```python
from build123d import *

# Parameters (mm, degrees)
SKETCH023_W  = 3.3
SKETCH023_H  = 2.2
PAD017_DEPTH = 2.5
PAD016_DEPTH = 5.5
FILLET001_R  = 1.1


with BuildPart() as pad_button_hole:
    # Sketch023 → Pad017 (new body)
    with BuildSketch(Plane.XY):
        Rectangle(SKETCH023_W, SKETCH023_H)
    extrude(amount=PAD017_DEPTH)


with BuildPart() as cut_button_small_final:
    # Sketch020 → Pad016 (new body)
    with BuildSketch(Plane.XY):
        with BuildLine():
            ThreePointArc((4.169285, 2.5), (0, 2.670418), (-4.169285, 2.5))
            ThreePointArc((-4.169285, 2.5), (-5.113877, 2.040693), (-5.5, 1.0639))
            ThreePointArc((-5.5, 1.0639), (-5.502959, 0), (-5.5, -1.0639))
            ThreePointArc((-5.5, -1.0639), (-5.113877, -2.040693), (-4.169285, -2.5))
            ThreePointArc((-4.169285, -2.5), (0, -2.670418), (4.169285, -2.5))
            ThreePointArc((4.169285, -2.5), (5.113877, -2.040693), (5.5, -1.0639))
            ThreePointArc((5.5, -1.0639), (5.502959, 0), (5.5, 1.0639))
            ThreePointArc((5.5, 1.0639), (5.113877, 2.040693), (4.169285, 2.5))
        make_face()
    extrude(amount=PAD016_DEPTH)

    # Fillet001
    fillet001_edges = [cut_button_small_final.edges().sort_by_distance(p)[0] for p in [
        (0, 2.670418, 5.5),
        (-5.113877, 2.040693, 5.5),
        (-5.502959, 0, 5.5),
        (-5.113877, -2.040693, 5.5),
        (0, -2.670418, 5.5),
        (5.113877, -2.040693, 5.5),
        (5.502959, 0, 5.5),
        (5.113877, 2.040693, 5.5),
    ]]
    fillet(fillet001_edges, radius=FILLET001_R)

    # Cut003: cut Pad (button hole)
    add(pad_button_hole.part, mode=Mode.SUBTRACT)


solid = cut_button_small_final.part
```
Source: CAD feature listing. Evaluate the final solid. Frame: model axes, mm. Round coordinates to 2 decimals unless told otherwise and drop trailing zeros. Loops run counter-clockwise (first coordinate to the right, second up) from the corner with the lowest first, then second, coordinate; pieces in that order, holes last.
1. Mould query, pull axis Y, two halves, no side actions, for faces 1 (the flat face through (0, 0, 2.5)), 2 (the cylindrical face through (-5.124, -2.03, 2.169)), 3 (the cylindrical face through (-5.104, 2.052, 2.169)). Classes: released by +Y, released by -Y, zero draft, split by the parting line, or undercut.
2. Ray query, L1, parallel to Y at x = 0.5, z = 1.15; L2, parallel to X at y = -0.5, z = 2; L3, parallel to Y at x = 0.5, z = 3.6. Return the intervals inside material, ascending.
3. Section query A-A on z = 0.8. Output: boundary loops of the cut face in (x, y).
4. Section query B-B on z = 3.95. Output: boundary loops of the cut face in (x, y).
5. Contact query for flat-ended pins moving along their axis: pin 1 (1.5 mm diameter, centred on x = 2.5, z = 4.5, fed in from +Y); pin 2 (1.1 mm diameter, centred on x = -0.5, y = 0.5, fed in from -Z). Output: stop coordinate, or through.
Answers below:
1. face 1: undercut
1. face 2: released by -Y
1. face 3: released by +Y
2. L1: y = -2.67 to -1.1, 1.1 to 2.67
2. L2: x = -5.5 to -1.65, 1.65 to 5.5
2. L3: y = -2.67 to 2.67
3. outline: (-5.5, -1.06) arc R1.45 ccw to (-4.17, -2.5) arc R51.09 ccw to (4.17, -2.5) arc R1.45 ccw to (5.5, -1.06) arc R191.26 ccw to (5.5, 1.06) arc R1.45 ccw to (4.17, 2.5) arc R51.09 ccw to (-4.17, 2.5) arc R1.45 ccw to (-5.5, 1.06) arc R191.26 ccw to start; hole (-1.65, -1.1) - (1.65, -1.1) - (1.65, 1.1) - (-1.65, 1.1) - close
4. outline: (-5.5, -1.06) arc R1.45 ccw to (-4.17, -2.5) arc R51.09 ccw to (4.17, -2.5) arc R1.45 ccw to (5.5, -1.06) arc R191.26 ccw to (5.5, 1.06) arc R1.45 ccw to (4.17, 2.5) arc R51.09 ccw to (-4.17, 2.5) arc R1.45 ccw to (-5.5, 1.06) arc R191.26 ccw to start
5. pin 1: stops at y = 2.64
5. pin 2: stops at z = 2.5
